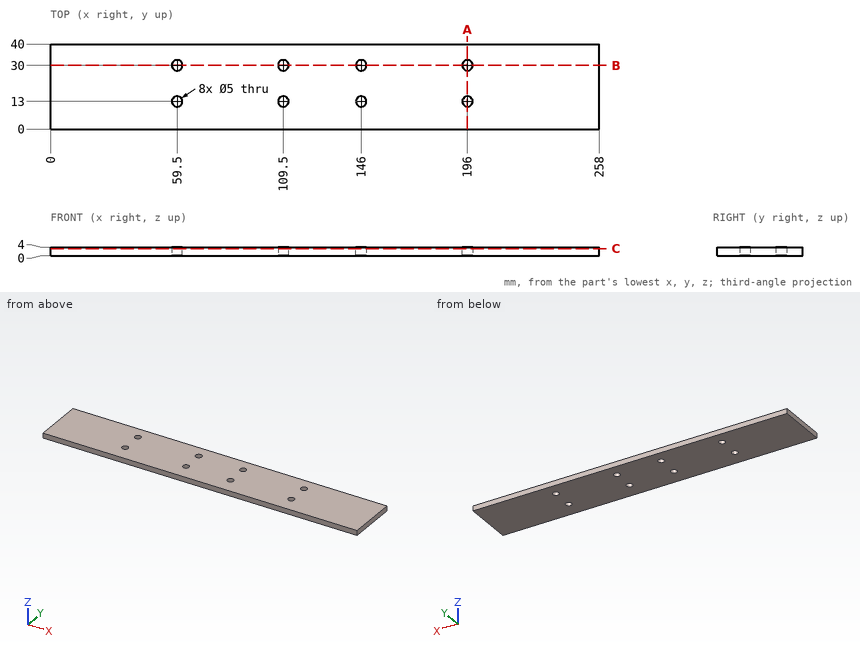
Job drawing, mm, ordinate dimensions from the low corner. One solid piece. Round coordinates to 2 decimals unless told otherwise and drop trailing zeros. Order: outer loops, then holes, each group sorted by start corner. A loop starts at its lowest first (then second) coordinate and runs counter-clockwise, first axis right, second up. Notation, with made-up numbers: (66, 44) -> (96, 44) arc R12 ccw to (96, 67) -> close; hole circle Ø5 at (-4, 16.5). An arc over 180 degrees is marked (long way). Answer in a Markdown table with one row per item.
1) Band-saw the part on A-A on x = 196. Give the cut face in (y, z).
Values:
| item | result |
|---|---|
| outline | (0, 0) -> (10.5, 0) -> (10.5, 4) -> (0, 4) -> close; (15.5, 0) -> (27.5, 0) -> (27.5, 4) -> (15.5, 4) -> close; (32.5, 0) -> (40, 0) -> (40, 4) -> (32.5, 4) -> close |
2) Band-saw the part on B-B on y = 30. Give the cut face in (x, z).
Values:
| item | result |
|---|---|
| outline | (0, 0) -> (57, 0) -> (57, 4) -> (0, 4) -> close; (62, 0) -> (107, 0) -> (107, 4) -> (62, 4) -> close; (112, 0) -> (143.5, 0) -> (143.5, 4) -> (112, 4) -> close; (148.5, 0) -> (193.5, 0) -> (193.5, 4) -> (148.5, 4) -> close; (198.5, 0) -> (258, 0) -> (258, 4) -> (198.5, 4) -> close |
3) Band-saw the part on C-C on z = 3.25. Give the number of separate pieces and of enclosed holes in the cut face, and give its area (3 significant figures).
Values:
| item | result |
|---|---|
| separate pieces | 1 |
| enclosed holes | 8 |
| area | 10,200 mm2 |
4) Wall check: L1, parallel to Y at x = 146, z = 2.7; L2, parallel to X at y = 13.5, z = 3; L3, parallel to X at y = 29, z = 3.2. Give the ranges that are in metal, low to high.
Values:
| item | result |
|---|---|
| L1 | 0 to 10.5, 15.5 to 27.5, 32.5 to 40 |
| L2 | 0 to 57.05, 61.95 to 107.05, 111.95 to 143.55, 148.45 to 193.55, 198.45 to 258 |
| L3 | 0 to 57.21, 61.79 to 107.21, 111.79 to 143.71, 148.29 to 193.71, 198.29 to 258 |
